The listing builds one solid part. Answer for the finished solid, in the listing's coordinates (mm). Face numbers are marked on the shaded views. A direction names the side the tool comes from. Give positions to 0.01 mm unless a question says otherwise; leave off trailing zeros. Order: outer loops, then holes, each group sorted by start corner. A loop starts at its lowest first (then second) coordinate and runs counter-clockwise, first axis right, second up. Notation, with made-up numbers: (41, 87) - (53, 87) arc R18 cw to (53, 94) - close; hole circle Ø3 at (51, 48.5). An arc over 180 degrees is marked (long way). Answer as a JSON object with one key per item and string values. Group by question number.
Q1. A cutting plane is placed at D-D, the plane y = 0. Give the vertices of the cut face in (x, z).
Q2. A cutting plane is placed at B-B, the plane x = 59. Give the vertices of the cut face in (y, z), and give its area (3 significant figures).
Q3. A cutting plane is placed at C-C, the plane z = 54.5. Give the vertices of the cut face in (x, y).
Q4. A cutting plane is placed at A-A, the plane z = 40. Give the vertices of the cut face in (x, y).
Q5. Consider line 1 (Z direction, x = 60, y = 5); line 2 (Y direction, x = 48.5, z = 68.5); line 3 (Y direction, x = 13, z = 49.5). Determine where each line is inside the solid, lowest interval first.
Q6. The mould has two halves that part along X. Classify the marked faces 1, 2 and 3: released by +X, released by -X, zero draft, split by the parting line, or undercut.
Q7. For the marked faces 4, 5 and 6, determine the directions among +Z, -Z, +X, -X, +Y, -Y from which every point of the face is accessible in a straight line to the end or side of a thin tool.
Q8. Given pin 1 (6 mm diameter, centred on x = 44.5, z = 66, fed in from -Y); pin 2 (3 mm diameter, centred on y = 13.5, z = 44, fed in from +X); pin 3 (6 mm diameter, centred on x = 47, z = 42.5, fed in from +Y), each flat-ended and moving along its own axis, determine where each tip first touches the part or whether it passes through.
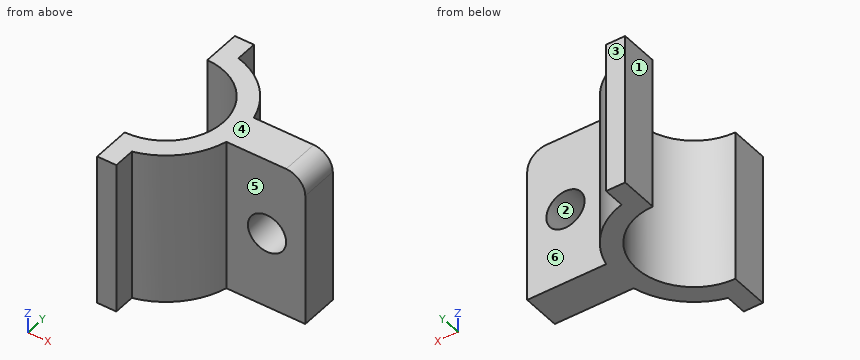
from build123d import *

# Parameters (mm, degrees)
EXTRUDE_1_DEPTH     = 80
SKETCH_2_R          = 10
CUT_EXTRUDE_1_DEPTH = 129.062484749
FILLET_1_R          = 10


with BuildPart() as part:
    # 草圖1 → 填料-伸長1 (new body)
    with BuildSketch(Plane.XY):
        with BuildLine():
            Line((0, -30), (0, -50))
            Line((0, -50), (10, -50))
            Line((10, -50), (10, -38.729833462))
            ThreePointArc((10, -38.729833462), (28.284271247, -28.284271247), (38.729833462, -10))
            Line((38.729833462, -10), (80, -10))
            Line((80, -10), (80, 10))
            Line((80, 10), (38.729833462, 10))
            ThreePointArc((38.729833462, 10), (28.284271247, 28.284271247), (10, 38.729833462))
            Line((10, 38.729833462), (10, 50))
            Line((10, 50), (0, 50))
            Line((0, 50), (0, 30))
            ThreePointArc((0, 30), (30, 0), (0, -30))
        make_face()
    extrude(amount=EXTRUDE_1_DEPTH)

    # 草圖2 → 除料-伸長1 (cut, through all)
    with BuildSketch(Plane.XZ.offset(10)):
        with Locations((60, 40)):
            Circle(SKETCH_2_R)
    extrude(amount=-CUT_EXTRUDE_1_DEPTH, mode=Mode.SUBTRACT)

    # 圓角1
    fillet_1_edges = [part.edges().sort_by_distance(p)[0] for p in [
        (80, 0, 80),
    ]]
    fillet(fillet_1_edges, radius=FILLET_1_R)


solid = part.part
Reply:
{
 "1": {"outline": "(30, 0) - (80, 0) - (80, 70) arc R10 ccw to (70, 80) - (30, 80) - close; hole circle Ø20 at (60, 40)"},
 "2": {"outline": "(-10, 0) - (10, 0) - (10, 30.05) - (-10, 30.05) - close; (-10, 49.95) - (10, 49.95) - (10, 80) - (-10, 80) - close", "area": "1,200 mm^2"},
 "3": {"outline": "(0, -50) - (10, -50) - (10, -38.73) arc R40 ccw to (38.73, -10) - (80, -10) - (80, 10) - (38.73, 10) arc R40 ccw to (10, 38.73) - (10, 50) - (0, 50) - (0, 30) arc R30 cw to (0, -30) - close"},
 "4": {"outline": "(0, -50) - (10, -50) - (10, -38.73) arc R40 ccw to (38.73, -10) - (50, -10) - (50, 10) - (38.73, 10) arc R40 ccw to (10, 38.73) - (10, 50) - (0, 50) - (0, 30) arc R30 cw to (0, -30) - close; (70, -10) - (80, -10) - (80, 10) - (70, 10) - close"},
 "5": {"line 1": "z = 0 to 30, 50 to 80", "line 2": "y = -10 to 10", "line 3": "y = -37.83 to -27.04, 27.04 to 37.83"},
 "6": {"face 1": "released by -X", "face 2": "undercut", "face 3": "zero draft"},
 "7": {"face 4": "+Z, +X, -X, +Y, -Y", "face 5": "+Z, -Z, +X, -Y", "face 6": "+Z, -Z, +X, +Y"},
 "8": {"pin 1": "stops at y = -10", "pin 2": "stops at x = 38.16", "pin 3": "stops at y = 10"}
}
